Geometry: final body of the model. Coordinates: model frame, mm. Face numbers are marked on the shaded views. A direction names the side the tool comes from. Round coordinates to 2 decimals unless told otherwise and drop trailing zeros. Loops run counter-clockwise (first coordinate to the right, second up) from the corner with the lowest first, then second, coordinate; pieces in that order, holes last. Notation, with made-up numbers: (-6.5, -28.5) - (50.5, -28.5) arc R19 ccw to (50.5, -22.5) - close; hole circle Ø5 at (43.5, -29). An arc over 180 degrees is marked (long way). Answer as CSV lines item,"result".
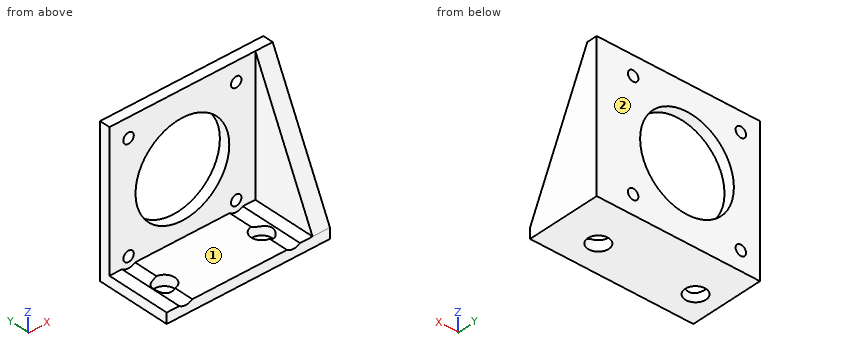
from build123d import *

# Parameters (mm, degrees)
SKETCH1_W           = 42
SKETCH1_H           = 21.3
BOSS_EXTRUDE1_DEPTH = 3
SKETCH2_R           = 3
CUT_EXTRUDE1_DEPTH  = 3
SKETCH4_W           = 42
SKETCH4_H           = 42
SKETCH4_R           = 1.5
SKETCH4_R_2         = 13.5
BOSS_EXTRUDE2_DEPTH = 3
BOSS_EXTRUDE3_DEPTH = 5
SKETCH6_R           = 3.134349401
CUT_EXTRUDE2_DEPTH  = 20


with BuildPart() as part:
    # Sketch1 → Boss-Extrude1 (new body)
    with BuildSketch(Plane.XY):
        with Locations((98.144783915, 168.215968794)):
            Rectangle(SKETCH1_W, SKETCH1_H)
    extrude(amount=BOSS_EXTRUDE1_DEPTH)

    # Sketch2 → Cut-Extrude1 (cut)
    with BuildSketch(Plane.XY.offset(3)):
        with Locations((112.144783915, 166.065968794)):
            Circle(SKETCH2_R)
        with Locations((84.144783915, 166.065968794)):
            Circle(SKETCH2_R)
    extrude(amount=-CUT_EXTRUDE1_DEPTH, mode=Mode.SUBTRACT)

    # Sketch4 → Boss-Extrude2 (add)
    with BuildSketch(Plane(origin=(0, 178.865968794, 0), x_dir=(-1, 0, 0), z_dir=(0, 1, 0))):
        with Locations((-98.144783915, 21)):
            Rectangle(SKETCH4_W, SKETCH4_H)
        with Locations((-113.644783915, 36.500179206)):
            Circle(SKETCH4_R, mode=Mode.SUBTRACT)
        with Locations((-82.644783915, 36.500179206)):
            Circle(SKETCH4_R, mode=Mode.SUBTRACT)
        with Locations((-82.644783915, 5.500179206)):
            Circle(SKETCH4_R, mode=Mode.SUBTRACT)
        with Locations((-113.644783915, 5.500179206)):
            Circle(SKETCH4_R, mode=Mode.SUBTRACT)
        with Locations((-98.144783915, 21.000179206)):
            Circle(SKETCH4_R_2, mode=Mode.SUBTRACT)
    extrude(amount=-BOSS_EXTRUDE2_DEPTH)

    # Sketch5 → Boss-Extrude3 (add)
    with BuildSketch(Plane(origin=(119.144783915, 0, 0), x_dir=(0, 0, -1), z_dir=(1, 0, 0))):
        Polygon((0, 157.565968794), (0, 178.865968794), (-42, 178.865968794), (-42, 175.865968794), (-3, 157.565968794), align=None)
    extrude(amount=BOSS_EXTRUDE3_DEPTH)

    # Sketch6 → Cut-Extrude2 (cut)
    with BuildSketch(Plane.XZ.offset(-175.865968794)):
        with Locations((82.644783915, 5.500179206)):
            Circle(SKETCH6_R)
        with Locations((113.644783915, 5.500179206)):
            Circle(SKETCH6_R)
    extrude(amount=CUT_EXTRUDE2_DEPTH, mode=Mode.SUBTRACT)


solid = part.part
(1) Pin query (flat end, axial travel): P1, Ø1.8, axis at x = 117.5, y = 164, coming from the +Z side; P2, Ø3.5, axis at x = 82.64, z = 36.5, coming from the -Y side; P3, Ø5.5, axis at y = 163, z = 16, coming from the -X side. Return the tip coordinate at first contact, or that it passes through.
Findings below:
P1,"z = 3"
P2,"y = 175.87"
P3,"x = 119.14"
(2) Section A-A (x = 88). Output: boundary loops of the cut face in (y, z).
Findings below:
outline,"(157.57, 0) - (178.87, 0) - (178.87, 12.09) - (175.87, 12.09) - (175.87, 3) - (157.57, 3) - close; (175.87, 29.91) - (178.87, 29.91) - (178.87, 42) - (175.87, 42) - close"
(3) Section C-C (z = 25). Output: boundary loops of the cut face in (x, y).
Findings below:
outline,"(77.14, 175.87) - (85.25, 175.87) - (85.25, 178.87) - (77.14, 178.87) - close; (111.04, 175.87) - (119.14, 175.87) - (119.14, 167.89) - (124.14, 167.89) - (124.14, 178.87) - (111.04, 178.87) - close"
(4) Material intervals for line 1 along Z through (x, y) = (90, 159.5); line 2 along Y through (x, z) = (87, 12.5); line 3 along X through (y, z) = (177, 33.5), sorted ascending.
Findings below:
line 1,"0 to 3"
line 2,"175.87 to 178.87"
line 3,"77.14 to 93.05, 103.24 to 124.14"
(5) Section D-D (y = 172.5). Output: boundary loops of the cut face in (x, z).
Findings below:
outline,"(77.14, 0) - (124.14, 0) - (124.14, 34.83) - (119.14, 34.83) - (119.14, 3) - (115.54, 3) arc R3.13 cw to (111.75, 3) - (84.54, 3) arc R3.13 cw to (80.75, 3) - (77.14, 3) - close"
(6) Section B-B (y = 165). Output: boundary loops of the cut face in (x, z), and give its area (3 significant figures).
Findings below:
outline,"(77.14, 0) - (81.34, 0) - (81.34, 2.65) arc R3.13 cw to (80.75, 3) - (77.14, 3) - close; (86.95, 0) - (109.34, 0) - (109.34, 3) - (86.95, 3) - close; (114.95, 0) - (124.14, 0) - (124.14, 18.84) - (119.14, 18.84) - (119.14, 3) - (115.54, 3) arc R3.13 cw to (114.95, 2.65) - close"
area,"186 mm2"
(7) Access query for the marked faces 1 and 2. Directions: +Z, -Z, +X, -X, +Y, -Y. A direction counts if a zero-diameter tool reaches every point of the face in a straight line with its end or side. Return the directions, or none.
Findings below:
face 1,"+Z, -X, -Y"
face 2,"+Z, -Z, +X, -X, +Y"
